For this review, use the dimensioned drawing (mm, ordinates from the lowest corner) and the shaded views. A direction names the side the tool comes from. Round coordinates to 2 decimals unless told otherwise and drop trailing zeros. Write each loop counter-clockwise with the first axis right and the second up, starting at its lowest first coordinate (ties: lowest second). Pieces come first, ordered by that corner, then holes.
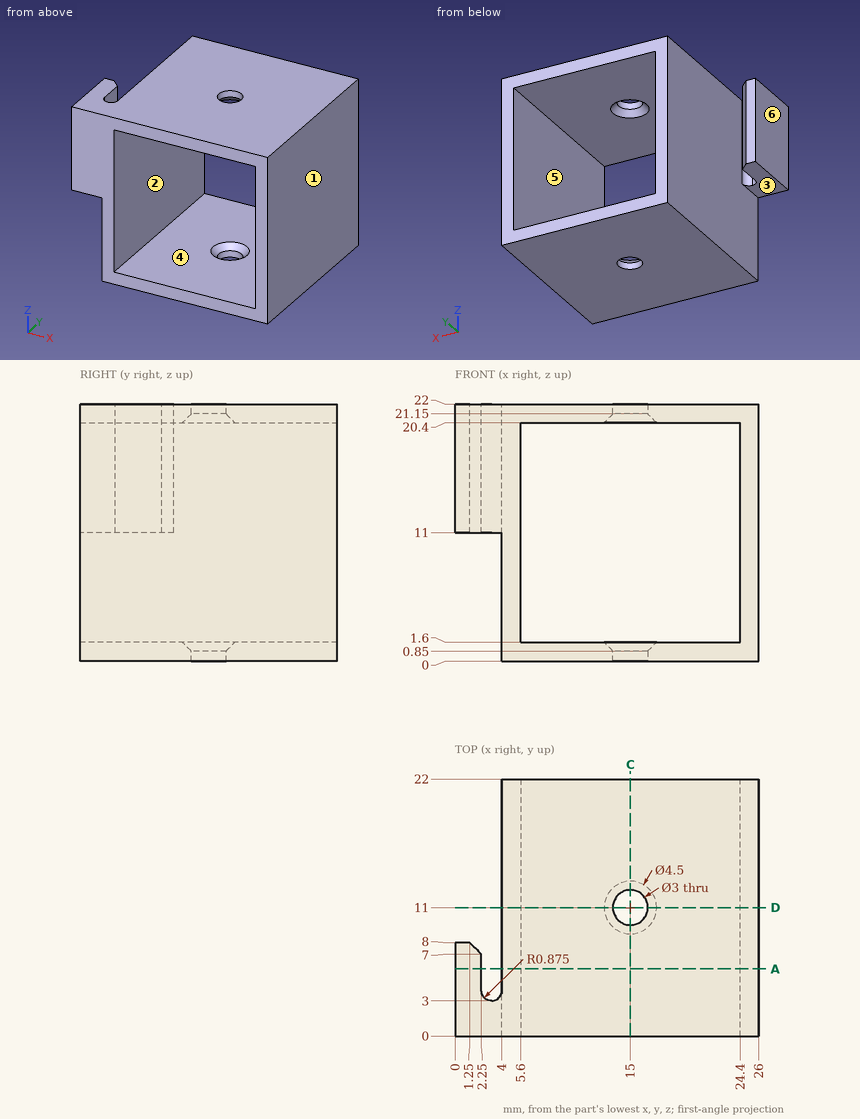
(1) We need section A-A, the plane y = 5.75. Give the boundary of the cut face in (x, z), and give its area (3 significant figures).
Geometry check:
outline: (0, 11) - (2.25, 11) - (2.25, 22) - (0, 22) - close; (4, 0) - (26, 0) - (26, 22) - (4, 22) - close; hole (5.6, 1.6) - (24.4, 1.6) - (24.4, 20.4) - (5.6, 20.4) - close
area: 155 mm2
(2) Mouldability with a two-part tool opening along Z and no side actions: class the marked faces 1, 2, 3 and 4 as pulls with the +Z half, pulls with the -Z half, needs draft (parallel to the pull), parting line crosses it, or undercut.
Geometry check:
face 1: needs draft
face 2: undercut
face 3: pulls with the -Z half
face 4: undercut
(3) We need section C-C, the plane x = 15. Give the boundary of the cut face in (y, z), and give its area (3 significant figures).
Geometry check:
outline: (0, 0) - (9.5, 0) - (9.5, 0.85) - (8.75, 1.6) - (0, 1.6) - close; (0, 20.4) - (8.75, 20.4) - (9.5, 21.15) - (9.5, 22) - (0, 22) - close; (12.5, 0) - (22, 0) - (22, 1.6) - (13.25, 1.6) - (12.5, 0.85) - close; (12.5, 21.15) - (13.25, 20.4) - (22, 20.4) - (22, 22) - (12.5, 22) - close
area: 59.7 mm2
(4) For the marked faces 5 and 6, list the 3-axis set-ups (+Z, -Z, +X, -X, +Y, -Y) from which the entire face can be reached by the end or side of a thin tool; tool diameter is ignored.
Geometry check:
face 5: +Y, -Y
face 6: +Z, -Z, -X, +Y, -Y
(5) For pin 1 Ø4 at (x, y) = (20.5, 8.5) entering from -Z; pin 2 Ø4 at (y, z) = (17, 11.5) entering from -X; pin 3 Ø1 at (x, z) = (1, 18.5) entering from +Y; pin 4 Ø1.2 at (x, y) = (1, 6) entering from -Z, all flat-tipped, find the tip position at first contact; note any pin that passes through.
Geometry check:
pin 1: stops at z = 0
pin 2: stops at x = 4
pin 3: stops at y = 8
pin 4: stops at z = 11
(6) For line 1 along Z through (x, y) = (15.5, 4.25); line 2 along X through (y, z) = (14, 8.5); line 3 along X through (y, z) = (1.25, 14), list the stretches that pass through material, from the lowest coordinate up.
Geometry check:
line 1: z = 0 to 1.6, 20.4 to 22
line 2: x = 4 to 5.6, 24.4 to 26
line 3: x = 0 to 5.6, 24.4 to 26
(7) We need section D-D, the plane y = 11. Give the boundary of the cut face in (x, z), and give its area (3 significant figures).
Geometry check:
outline: (4, 0) - (13.5, 0) - (13.5, 0.85) - (12.75, 1.6) - (5.6, 1.6) - (5.6, 20.4) - (12.75, 20.4) - (13.5, 21.15) - (13.5, 22) - (4, 22) - close; (16.5, 0) - (26, 0) - (26, 22) - (16.5, 22) - (16.5, 21.15) - (17.25, 20.4) - (24.4, 20.4) - (24.4, 1.6) - (17.25, 1.6) - (16.5, 0.85) - close
area: 120 mm2
